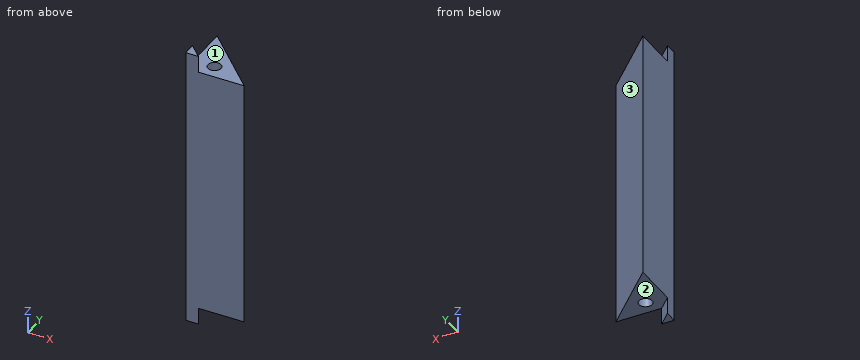
from build123d import *

# Parameters (mm, degrees)
RESSALTO_EXTRUS_O1_DEPTH                    = 60
RESSALTO_EXTRUS_O2_DEPTH                    = 4
RESSALTO_EXTRUS_O3_DEPTH                    = 4
FURO_ROSCADO_PARA_CONDU_TE_DE_M3X0_51_D     = 3.15
FURO_ROSCADO_PARA_CONDU_TE_DE_M3X0_51_DEPTH = 10
FURO_ROSCADO_PARA_CONDU_TE_DE_M3X0_51_TIP   = 0.946355475
FURO_ROSCADO_PARA_CONDU_TE_DE_M3X0_52_D     = 3.15
FURO_ROSCADO_PARA_CONDU_TE_DE_M3X0_52_DEPTH = 7.5
FURO_ROSCADO_PARA_CONDU_TE_DE_M3X0_52_TIP   = 0.946355475


with BuildPart() as part:
    # Esboço1 → Ressalto-extrusão1 (new body)
    with BuildSketch(Plane.XY):
        Polygon((0, 0), (14, 0), (0, 14), align=None)
    extrude(amount=RESSALTO_EXTRUS_O1_DEPTH)

    # Esboço2 → Ressalto-extrusão2 (add)
    with BuildSketch(Plane.XY.offset(60)):
        Polygon((0, 0), (0, 3), (3, 0), align=None)
    extrude(amount=RESSALTO_EXTRUS_O2_DEPTH)

    # Esboço3 → Ressalto-extrusão3 (add)
    with BuildSketch(Plane(origin=(0, 0, 0), x_dir=(-1, 0, 0), z_dir=(0, 0, -1))):
        Polygon((0, 0), (0, 3), (-3, 0), align=None)
    extrude(amount=RESSALTO_EXTRUS_O3_DEPTH)

    # Furo roscado para conduíte de M3x0.51
    with Locations(Plane.XY.offset(60)):
        with Locations((5, 3.5)):
            Hole(FURO_ROSCADO_PARA_CONDU_TE_DE_M3X0_51_D / 2, depth=FURO_ROSCADO_PARA_CONDU_TE_DE_M3X0_51_DEPTH)
            with Locations((0, 0, -(FURO_ROSCADO_PARA_CONDU_TE_DE_M3X0_51_DEPTH + FURO_ROSCADO_PARA_CONDU_TE_DE_M3X0_51_TIP / 2))):  # 118° drill point
                Cone(0, FURO_ROSCADO_PARA_CONDU_TE_DE_M3X0_51_D / 2, FURO_ROSCADO_PARA_CONDU_TE_DE_M3X0_51_TIP, mode=Mode.SUBTRACT)

    # Furo roscado para conduíte de M3x0.52
    with Locations(Plane(origin=(0, 0, 0), x_dir=(-1, 0, 0), z_dir=(0, 0, -1))):
        with Locations((-5, 3.5)):
            Hole(FURO_ROSCADO_PARA_CONDU_TE_DE_M3X0_52_D / 2, depth=FURO_ROSCADO_PARA_CONDU_TE_DE_M3X0_52_DEPTH)
            with Locations((0, 0, -(FURO_ROSCADO_PARA_CONDU_TE_DE_M3X0_52_DEPTH + FURO_ROSCADO_PARA_CONDU_TE_DE_M3X0_52_TIP / 2))):  # 118° drill point
                Cone(0, FURO_ROSCADO_PARA_CONDU_TE_DE_M3X0_52_D / 2, FURO_ROSCADO_PARA_CONDU_TE_DE_M3X0_52_TIP, mode=Mode.SUBTRACT)


solid = part.part
Can you work these out from the model? Positions are in its coordinate system, mm. Face numbers are marked on the shaded views. A direction names the side the tool comes from. Give positions to 0.01 mm unless a question says otherwise; leave off trailing zeros. Order: outer loops, then holes, each group sorted by start corner. A loop starts at its lowest first (then second) coordinate and runs counter-clockwise, first axis right, second up. Notation, with made-up numbers: M 14,62 L 52,62 A29 ccw 52,89 Z; hole C 33,-13.5 d5. An arc over 180 degrees is marked long. One line per question, with ' | ' between items.
Item 1: For the marked faces 1, 2 and 3, which set-ups out of +Z, -Z, +X, -X, +Y, -Y let a thin tool reach every point of the face, with its end or its side?
Answer block:
face 1: +Z, +X, +Y | face 2: -Z, +X, +Y | face 3: +Z, -Z, +X, +Y
Item 2: I'm going to push flat-ended pins straight in: pin 1 Ø5 at (x, y) = (6.5, 1.5) entering from -Z; pin 2 Ø5 at (y, z) = (9.5, 26) entering from +X; pin 3 Ø3 at (y, z) = (10, 42) entering from +X. Where does each tip first touch, or does it pass through?
Answer block:
pin 1: stops at z = 0 | pin 2: stops at x = 7 | pin 3: stops at x = 5.5
Item 3: Suppose I cut it at B-B, the plane y = 7. Write out the boundary of the cut face in (x, z).
Answer block:
outline: M 0,0 L 7,0 L 7,60 L 0,60 Z
Item 4: Suppose I cut it at C-C, the plane z = 20. Write out the boundary of the cut face in (x, y), then the cut area to 3 significant figures.
Answer block:
outline: M 0,0 L 14,0 L 0,14 Z | area: 98.0 mm2
Item 5: Please list where these lines run through material, in increasing order: L1, parallel to Z at x = 5.75, y = 5.25; L2, parallel to Y at x = 5, z = 3.5 (3 decimals); L3, parallel to Y at x = 6, z = 6.5.
Answer block:
L1: z = 0 to 60 | L2: y = 0 to 1.925, 5.075 to 9 | L3: y = 0 to 2.28, 4.72 to 8
Item 6: Suppose I cut it at D-D, the plane y = 11.5. Write out the boundary of the cut face in (x, z).
Answer block:
outline: M 0,0 L 2.5,0 L 2.5,60 L 0,60 Z
Item 7: Suppose I cut it at A-A, the plane x = 2.25. Write out the boundary of the cut face in (y, z).
Answer block:
outline: M 0,-4 L 0.75,-4 L 0.75,0 L 11.75,0 L 11.75,60 L 0.75,60 L 0.75,64 L 0,64 Z
